Source: CAD feature listing. Evaluate the final solid. Frame: model axes, mm. A direction names the side the tool comes from. Give positions to 0.01 mm unless a question says otherwise; leave off trailing zeros. Loops run counter-clockwise (first coordinate to the right, second up) from the corner with the lowest first, then second, coordinate; pieces in that order, holes last. Notation, with made-up numbers: (5.25, 31.5) - (35.25, 31.5) arc R33 ccw to (35.25, 67.5) - close; hole circle Ø10 at (44, 4.5). An arc over 180 degrees is marked (long way). Put each result on its own line as item: value.
Autodesk Inventor part; units mm, degrees
ref_plane "YZ Plane" through (0, 0, 0) normal (1, 0, 0) x (0, 1, 0)
ref_plane "XZ Plane" through (0, 0, 0) normal (0, 1, 0) x (-1, 0, 0)
ref_plane "XY Plane" through (0, 0, 0) normal (0, 0, 1) x (1, 0, 0)
sketch "Boceto1" plane through (0, 0, 0) normal (0, 1, 0) x (-1, 0, 0)
  line L0 (45, 172) -> (-45, 172)
  line L1 (-45, 172) -> (-45, -172)
  line L2 (-45, -172) -> (45, -172)
  line L3 (45, -172) -> (45, 172)
  line L4 (45, 172) -> (-45, -172) construction
  line L5 (-45, 172) -> (45, -172) construction
  circle A0 centre (0, -172) radius 45
  circle A1 centre (0, 172) radius 45
  circle A2 centre (0, 172) radius 34.798
  line L6 (45, 172) -> (-45, 172)
  point P0 (0, 0)
  dimension "d0" = 90
  dimension "d1" = 344
  dimension "d2" = 90
  dimension "d3" = 90
  dimension "d4" = 69.596
extrude "Extrusión1" add sketch "Boceto1" along normal blind 20 contours A1 L0 A2 | L0 A2 A1 | L3 A0 L1 A1 | A2 L0 | A0 L2 | L2 A0 picked at (9.4719, 153.1181)
sketch "Boceto3" plane through (0, 20, 0) normal (0, 1, 0) x (1, 0, 0)
  line L0 (34.798, -172) -> (-34.798, -172)
  circle A0 centre (0, -172) radius 34.798
  point P0 (0, 0)
extrude "Extrusión2" cut sketch "Boceto3" against normal blind 20
sketch "Boceto5" plane through (0, 20, 0) normal (0, 1, 0) x (1, 0, 0)
  circle A0 centre (0, -172) radius 34.798
  line L0 (-45, 172) -> (-45, -172)
  arc A1 (-45, -172) -> (45, -172) centre (0, -172) ccw
  line L1 (45, -172) -> (45, 172)
  arc A2 (45, 172) -> (-45, 172) centre (0, 172) ccw
  line L2 (34.798, -172) -> (-34.798, 172) construction
  line L3 (-34.798, -172) -> (34.798, 172) construction
  line L4 (-45, 172) -> (-45, -172)
  arc A3 (34.798, -143.4676) -> (-34.798, -143.4676) centre (0, -172) ccw
  arc A4 (-34.798, 143.4676) -> (34.798, 143.4676) centre (0, 172) ccw
  line L5 (-34.798, -143.4676) -> (-34.798, 143.4676)
  line L6 (34.798, 143.4676) -> (34.798, -143.4676)
  line L7 (45, -172) -> (45, 172)
  point P0 (0, 0)
extrude "Extrusión3" cut sketch "Boceto5" against normal blind 20 contours A3 L5 A4 L6
sketch "Boceto6" plane through (0, 20, 0) normal (0, 1, 0) x (1, 0, 0)
  circle A0 centre (0, -172) radius 34.798
  arc A1 (34.798, -143.4676) -> (-34.798, -143.4676) centre (0, -172) ccw
  arc A2 (-45, -172) -> (45, -172) centre (0, -172) ccw
  arc A3 (-34.798, 143.4676) -> (34.798, 143.4676) centre (0, 172) ccw
  circle A4 centre (0, -172) radius 34.798
  circle A5 centre (0, -172) radius 45
  circle A6 centre (0, 172) radius 45
  point P0 (0, 0)
extrude "Extrusión4" add sketch "Boceto6" along normal blind 40.35 contours A5 A2 A1
chamfer "Chaflán1" distance 6.35 angle 45 2 edges at (-34.798, 60.35, 172) (34.798, 0, 172)
sketch "Boceto7" plane through (0, 20, 0) normal (0, 1, 0) x (1, 0, 0)
  arc A0 (-34.798, -143.4676) -> (-45, -172) centre (0, -172) ccw
  line L0 (-34.798, -143.4676) -> (-34.798, 143.4676)
  arc A1 (-34.798, 143.4676) -> (34.798, 143.4676) centre (0, 172) ccw
  line L1 (34.798, 143.4676) -> (34.798, -143.4676)
  arc A2 (45, -172) -> (34.798, -143.4676) centre (0, -172) ccw
  line L2 (45, -172) -> (45, 172)
  arc A3 (45, 172) -> (-45, 172) centre (0, 172) ccw
  line L3 (-45, 172) -> (-45, -172)
  circle A4 centre (0, 172) radius 30.48
  point P0 (0, 0)
  dimension "d16" = 60.96
extrude "Extrusión5" add sketch "Boceto7" along normal blind 88.9 contours A4
sketch "Boceto9" plane through (0, 108.9, -172) normal (0, 1, 0) x (1, 0, 0)
  circle A0 centre (0, 0) radius 36
  point P0 (0, -172)
  dimension "d20" = 72
extrude "Extrusión6" add sketch "Boceto9" against normal blind 30.48
chamfer "Chaflán2" distance 10.56 angle 45 1 edges at (-36, 108.9, -172)
chamfer "Chaflán3" distance 5.08 angle 45 1 edges at (-36, 78.42, -172)
fillet "Empalme1" radius 5 1 edges at (-30.48, 20, -172)
sketch "Boceto10" plane through (0, 108.9, -172) normal (0, 1, 0) x (1, 0, 0)
  circle A0 centre (0, 0) radius 25.44
  arc A1 (45, 0) -> (-45, 0) centre (0, 0) ccw
  line L0 (44.3276, -7.75) -> (-44.3276, -7.75)
  line L1 (-44.3276, -7.75) -> (-44.3276, 7.75)
  line L2 (-44.3276, 7.75) -> (44.3276, 7.75)
  line L3 (44.3276, 7.75) -> (44.3276, -7.75)
  line L4 (44.3276, -7.75) -> (-44.3276, 7.75) construction
  line L5 (-44.3276, -7.75) -> (44.3276, 7.75) construction
  point P0 (0, -172)
  dimension "d30" = 15.5
extrude "Extrusión7" cut sketch "Boceto10" against normal blind 88.9 contours A0 L0 L2 | A0 L2 L3 L0 | A0 L0 L1 L2
ref_plane "Plano de trabajo1" through (0, 0, -217) normal (0, 0, -1) x (-1, 0, 0)
sketch "Boceto11" plane through (0, 0, -217) normal (0, 0, -1) x (-1, 0, 0)
  line L0 (45, 0) -> (45, 20)
  line L1 (-45, 20) -> (45, 20)
  line L2 (-45, 20) -> (-45, 0)
  line L3 (-45, 0) -> (45, 0)
  line L4 (45, 0) -> (-45, 0)
  line L5 (-20, 20) -> (20, 20)
  line L6 (20, 20) -> (20, 0)
  line L7 (20, 0) -> (-20, 0)
  line L8 (-20, 0) -> (-20, 20)
  line L9 (-20, 20) -> (20, 0) construction
  line L10 (20, 20) -> (-20, 0) construction
  point P0 (0, 0)
  point P1 (0, 10)
extrude "Extrusión8" add sketch "Boceto11" along normal blind 30 and the other way blind 10 contours L3 L8 L1 L6
sketch "Boceto15" plane through (0, 20, 0) normal (0, 1, 0) x (1, 0, 0)
  arc A0 (-20, 212.3113) -> (-45, 172) centre (0, 172) ccw
  line L0 (-45, 172) -> (-45, -172)
  arc A1 (-34.798, -143.4676) -> (-45, -172) centre (0, -172) ccw
  line L1 (-34.798, -143.4676) -> (-34.798, 143.4676)
  arc A2 (-34.798, 143.4676) -> (34.798, 143.4676) centre (0, 172) ccw
  line L2 (34.798, 143.4676) -> (34.798, -143.4676)
  arc A3 (45, -172) -> (34.798, -143.4676) centre (0, -172) ccw
  line L3 (45, -172) -> (45, 172)
  arc A4 (45, 172) -> (20, 212.3113) centre (0, 172) ccw
  line L4 (20, 212.3113) -> (20, 247)
  line L5 (-20, 247) -> (20, 247)
  line L6 (-20, 212.3113) -> (-20, 247)
  arc A5 (34.6232, 179.75) -> (-34.6232, 179.75) centre (0, 172) ccw
  line L7 (-34.6232, 179.75) -> (34.6232, 179.75)
  line L8 (34.6232, 164.25) -> (-34.6232, 164.25)
  arc A6 (-34.6232, 164.25) -> (34.6232, 164.25) centre (0, 172) ccw
  arc A7 (12, 227) -> (-12, 227) centre (0, 227) ccw
  line L9 (12, 227) -> (12, 212.3113)
  line L10 (-12, 227) -> (-12, 212.3113)
  arc A8 (45, 172) -> (20, 212.3113) centre (0, 172) ccw
  line L11 (-20, 227) -> (-20, 247)
  line L12 (20, 247) -> (-20, 247)
  line L13 (-20, 247) -> (20, 247)
  line L14 (20, 247) -> (20, 227)
  line L15 (-12, 212.3113) -> (12, 212.3113)
  line L16 (-20, 227) -> (-20, 247)
  line L17 (20, 247) -> (0, 247)
  line L18 (-20, 247) -> (0, 247)
  line L19 (-20, 247) -> (-20, 227)
  arc A9 (20, 227) -> (0, 247) centre (0, 227) ccw
  arc A10 (0, 247) -> (-20, 227) centre (0, 227) ccw
  line L20 (20, 212.3113) -> (20, 247)
  line L21 (20, 227) -> (20, 247)
  line L22 (20, 247) -> (0, 247)
  point P0 (0, 0)
extrude "Extrusión11" cut sketch "Boceto15" against normal blind 50 contours L6 L5 A10 | L5 L4 A9 | L9 L15 L10 A7
sketch "Boceto16" plane through (20, 0, -212.3113) normal (1, 0, 0) x (0, 0, -1)
  line L0 (14.6887, 0) -> (14.6887, 20)
  line L1 (0, 20) -> (14.6887, 20)
  line L2 (0, 0) -> (0, 20)
  line L3 (0, 0) -> (14.6887, 0)
  line L4 (0, 20) -> (38, 20)
  line L5 (38, 20) -> (38, 9)
  line L6 (38, 9) -> (0, 9)
  line L7 (0, 9) -> (0, 20)
  point P0 (-212.3113, 0)
extrude "Extrusión12" cut sketch "Boceto16" against normal blind 50 contours L6 L2 L1 L0 | L0 L4 L5 L6
properties part number "link_v2ipt"
1) Material intervals for line 1 along Z through (x, y) = (0, 16.5); line 2 along X through (y, z) = (19, 172); line 3 along Z through (x, y) = (-21.5, 55.5), sorted ascending. Write a range as [from, to].
Check result:
line 1: [-212.31, -127], [127, 137.2], [206.8, 217]
line 2: [-45, -34.8], [34.8, 45]
line 3: [-193.61, -179.75], [-164.25, -150.39], [132.47, 142.75], [201.25, 211.53]
2) Mould query, pull axis Y, two halves, no side actions, for faces 1 (the flat face through (0, 9, -241)), 2 (the flat face through (-2.36, 78.42, -202.54)), 3 (the flat face through (-45, 10, -2)). Classes: pulls with the +Y half, pulls with the -Y half, needs draft (parallel to the pull), parting line crosses it, or undercut.
Check result:
face 1: pulls with the +Y half
face 2: undercut
face 3: needs draft
3) Section query C-C, the plane y = 36. Output: boundary loops of the cut face in (x, z), plus the area to 3 significant figures.
Check result:
outline: circle Ø90 at (0, 172); (-29.48, -179.75) arc R30.48 ccw to (29.48, -179.75) - close; (-29.48, -164.25) - (29.48, -164.25) arc R30.48 ccw to start; hole circle Ø69.6 at (0, 172)
area: 4,540 mm²
4) Section query D-D, the plane y = 14.5. Output: boundary loops of the cut face in (x, z).
Check result:
outline: (-45, -172) arc R45 ccw to (-20, -212.31) - (20, -212.31) arc R45 ccw to (45, -172) - (45, 172) arc R45 ccw to (-45, 172) - close; hole (-34.8, -143.47) arc R45 cw to (34.8, -143.47) - (34.8, 143.47) arc R45 cw to (-34.8, 143.47) - close; hole circle Ø69.6 at (0, 172)
5) Access query for faces 4 (the flat face through (0, 65, -164.25)), 5 (the flat face through (20, 4, -220)), 6 (the flat face through (-20, 5, -220)), 7 (the cylindrical face through (0, 5, -239)), 8 (the conical face through (-0.592, 78.738, -140.768)). Directions: +Z, -Z, +X, -X, +Y, -Y. A direction counts if a zero-diameter tool reaches every point of the face in a straight line with its end or side. Return the directions, or none.
Check result:
face 4: +X, -X, +Y
face 5: -Z, +X, +Y, -Y
face 6: -Z, -X, +Y, -Y
face 7: +Y, -Y
face 8: +Z
6) Pin query (flat end, axial travel): P1, Ø4.5, axis at y = 6, z = -216, coming from the +X side; P2, Ø2, axis at x = 34, y = 60, coming from the +Z side; P3, Ø10, axis at x = 27.5, z = -33.5, coming from the -Y side; P4, Ø6, axis at x = -7.5, y = 9, coming from the -Z side. Return the tip coordinate at first contact, or that it passes through.
Check result:
P1: x = 20
P2: z = 202.59
P3: through
P4: z = -246.49
7) Section query B-B, the plane z = 36.5. Output: boundary loops of the cut face in (x, y), plus the area to 3 significant figures.
Check result:
outline: (-45, 0) - (-34.8, 0) - (-34.8, 20) - (-45, 20) - close; (34.8, 0) - (45, 0) - (45, 20) - (34.8, 20) - close
area: 408 mm²
